```python
from build123d import *

# Parameters (mm, degrees)
ESBO_O1_W                = 300
ESBO_O1_H                = 200
RESSALTO_EXTRUS_O1_DEPTH = 500
ESBO_O2_W                = 296
ESBO_O2_H                = 196
CORTE_EXTRUS_O1_DEPTH    = 501
ESBO_O3_R                = 2
ESBO_O3_R_2              = 2.5
ESBO_O3_W                = 260
ESBO_O3_H                = 40
CORTE_EXTRUS_O2_DEPTH    = 10
ESBO_O5_R                = 2.5
CORTE_EXTRUS_O3_DEPTH    = 201


with BuildPart() as part:
    # Esboço1 → Ressalto-extrusão1 (new body)
    with BuildSketch(Plane(origin=(0, 0, 0), x_dir=(0, 0, -1), z_dir=(1, 0, 0))):
        Rectangle(ESBO_O1_W, ESBO_O1_H)
    extrude(amount=RESSALTO_EXTRUS_O1_DEPTH)

    # Esboço2 → Corte-extrusão1 (cut, through all)
    with BuildSketch(Plane(origin=(500, 0, 0), x_dir=(0, 0, -1), z_dir=(1, 0, 0))):
        Rectangle(ESBO_O2_W, ESBO_O2_H)
    extrude(amount=-CORTE_EXTRUS_O1_DEPTH, mode=Mode.SUBTRACT)

    # Esboço3 → Corte-extrusão2 (cut)
    with BuildSketch(Plane(origin=(0, 100, 0), x_dir=(1, 0, 0), z_dir=(0, 1, 0))):
        with Locations((57.5, 0)):
            Circle(ESBO_O3_R)
        with Locations((442.5, 0)):
            Circle(ESBO_O3_R)
        with Locations((120, 47.5)):
            Circle(ESBO_O3_R_2)
        with Locations((200, 47.5)):
            Circle(ESBO_O3_R_2)
        with Locations((300, 47.5)):
            Circle(ESBO_O3_R_2)
        with Locations((380, 47.5)):
            Circle(ESBO_O3_R_2)
        with Locations((380, -47.5)):
            Circle(ESBO_O3_R_2)
        with Locations((300, -47.5)):
            Circle(ESBO_O3_R_2)
        with Locations((200, -47.5)):
            Circle(ESBO_O3_R_2)
        with Locations((120, -47.5)):
            Circle(ESBO_O3_R_2)
        with Locations((250, 0)):
            Rectangle(ESBO_O3_W, ESBO_O3_H)
    extrude(amount=-CORTE_EXTRUS_O2_DEPTH, mode=Mode.SUBTRACT)

    # Esboço5 → Corte-extrusão3 (cut, through all)
    with BuildSketch(Plane(origin=(0, 100, 0), x_dir=(1, 0, 0), z_dir=(0, 1, 0))):
        with Locations((490, 130)):
            Circle(ESBO_O5_R)
        with Locations((490, 65)):
            Circle(ESBO_O5_R)
        with Locations((490, 0)):
            Circle(ESBO_O5_R)
        with Locations((490, -65)):
            Circle(ESBO_O5_R)
        with Locations((490, -130)):
            Circle(ESBO_O5_R)
        with Locations((10, -130)):
            Circle(ESBO_O5_R)
        with Locations((10, -65)):
            Circle(ESBO_O5_R)
        with Locations((10, 0)):
            Circle(ESBO_O5_R)
        with Locations((10, 65)):
            Circle(ESBO_O5_R)
        with Locations((10, 130)):
            Circle(ESBO_O5_R)
    extrude(amount=-CORTE_EXTRUS_O3_DEPTH, mode=Mode.SUBTRACT)


solid = part.part
```
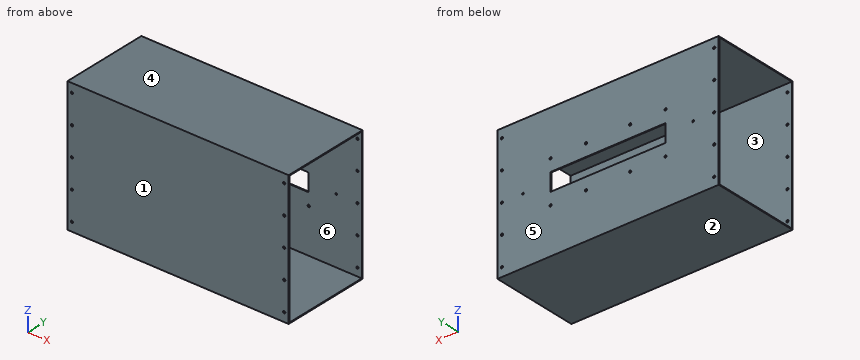
Build history of the part. All positions in model axes, mm. Face numbers are marked on the shaded views. A direction names the side the tool comes from. Round coordinates to 2 decimals unless told otherwise and drop trailing zeros. Write each loop counter-clockwise with the first axis right and the second up, starting at its lowest first coordinate (ties: lowest second). Pieces come first, ordered by that corner, then holes. Notation, with made-up numbers: (71, -19.75) - (126, -19.75) arc R20 cw to (126, 5.25) - close; hole circle Ø10 at (-26.75, 48). An arc over 180 degrees is marked (long way). Write each question's results on one line, items separated by ' | '. Start each with the question number.
Item 1: Drop flat-ended pins along their axis: P1, Ø4, axis at x = 490, z = 130, coming from the +Y side; P2, Ø1.5, axis at x = 217.5, z = 2, coming from the +Y side. Give the stop position or say it passes through.
Item 2: Saw through at B-B (x = 400.5). Write the cut outline in (y, z).
Item 3: Saw through at A-A (y = 51.5). Write the cut outline in (x, z), and give its area (3 significant figures).
Item 4: Wall check: L1, parallel to Z at x = 10, y = 98.4; L2, parallel to Z at x = 200, y = 98.7; L3, parallel to X at y = -98.85, z = 130. Give the ranges that are in metal, low to high. Write a range as [from, to].
Item 5: Which spindle directions (+Z, -Z, +X, -X, +Y, -Y) get a long thin tool onto all of the face, cutting with end or side? Do the marked faces 5 and 6. Say none if no direction does.
Item 6: Saw through at C-C (x = 266). Write the cut outline in (y, z).
Item 7: Mould opens along Z. For the marked faces 1, 2, 3 and 4 say: pulls with the +Z half, pulls with the -Z half, needs draft (parallel to the pull), parting line crosses it, or undercut.
Results are:
1) P1: passes through | P2: stops at y = -98
2) outline: (-100, -150) - (100, -150) - (100, 150) - (-100, 150) - close; hole (-98, -148) - (98, -148) - (98, 148) - (-98, 148) - close
3) outline: (0, -150) - (500, -150) - (500, -148) - (0, -148) - close; (0, 148) - (500, 148) - (500, 150) - (0, 150) - close | area: 2,000 mm²
4) L1: z = [-150, -132.5], [-127.5, -67.5], [-62.5, -2.5], [2.5, 62.5], [67.5, 127.5], [132.5, 150] | L2: z = [-150, -50], [-45, -20], [20, 45], [50, 150] | L3: x = [0, 7.5], [12.5, 487.5], [492.5, 500]
5) face 5: +Z, -Z, +X, -X, +Y | face 6: +X, -X
6) outline: (-100, -150) - (100, -150) - (100, -20) - (98, -20) - (98, -148) - (-98, -148) - (-98, 148) - (98, 148) - (98, 20) - (100, 20) - (100, 150) - (-100, 150) - close
7) face 1: needs draft | face 2: pulls with the -Z half | face 3: undercut | face 4: pulls with the +Z half
